from build123d import *

# Parameters (mm, degrees)
BOSS_EXTRUDE1_DEPTH        = 20
F_6_CLEARANCE_HOLE1_REACH  = 91.156
F_6_CLEARANCE_HOLE1_BORE_R = 1.89865
F_1_CLEARANCE_HOLE1_REACH  = 91.156
F_1_CLEARANCE_HOLE1_BORE_R = 1.0287
F_6_CLEARANCE_HOLE2_D      = 3.7973


with BuildPart() as part:
    # Sketch1 → Boss-Extrude1 (new body)
    with BuildSketch(Plane.XY):
        Polygon((30, 0), (0, 0), (0, 81.54), (30, 81.54), (30, 79.9525), (1.5875, 79.9525), (1.5875, 1.5875), (30, 1.5875), align=None)
    extrude(amount=BOSS_EXTRUDE1_DEPTH)

    # #6 Clearance Hole1 bore → #6 Clearance Hole1 (cut, up to next)
    with BuildSketch(Plane(origin=(0, 81.54, 0), x_dir=(1, 0, 0), z_dir=(0, 1, 0)), mode=Mode.PRIVATE) as f_6_clearance_hole1_sk1:
        with Locations((5, -10)):
            Circle(F_6_CLEARANCE_HOLE1_BORE_R)
    f_6_clearance_hole1_tool1 = extrude(f_6_clearance_hole1_sk1.sketch, amount=-F_6_CLEARANCE_HOLE1_REACH, mode=Mode.PRIVATE) & part.part
    # #6 Clearance Hole1 bore → #6 Clearance Hole1 (cut, up to next)
    with BuildSketch(Plane(origin=(0, 81.54, 0), x_dir=(1, 0, 0), z_dir=(0, 1, 0)), mode=Mode.PRIVATE) as f_6_clearance_hole1_sk2:
        with Locations((25, -10)):
            Circle(F_6_CLEARANCE_HOLE1_BORE_R)
    f_6_clearance_hole1_tool2 = extrude(f_6_clearance_hole1_sk2.sketch, amount=-F_6_CLEARANCE_HOLE1_REACH, mode=Mode.PRIVATE) & part.part
    add(f_6_clearance_hole1_tool1.solids().sort_by_distance((5, 81.54, 10))[0], mode=Mode.SUBTRACT)
    add(f_6_clearance_hole1_tool2.solids().sort_by_distance((25, 81.54, 10))[0], mode=Mode.SUBTRACT)

    # #1 Clearance Hole1 bore → #1 Clearance Hole1 (cut, up to next)
    with BuildSketch(Plane(origin=(0, 0, 0), x_dir=(-1, 0, 0), z_dir=(0, -1, 0)), mode=Mode.PRIVATE) as f_1_clearance_hole1_sk1:
        with Locations((-5.9, -10)):
            Circle(F_1_CLEARANCE_HOLE1_BORE_R)
    f_1_clearance_hole1_tool1 = extrude(f_1_clearance_hole1_sk1.sketch, amount=-F_1_CLEARANCE_HOLE1_REACH, mode=Mode.PRIVATE) & part.part
    # #1 Clearance Hole1 bore → #1 Clearance Hole1 (cut, up to next)
    with BuildSketch(Plane(origin=(0, 0, 0), x_dir=(-1, 0, 0), z_dir=(0, -1, 0)), mode=Mode.PRIVATE) as f_1_clearance_hole1_sk2:
        with Locations((-24.1, -10)):
            Circle(F_1_CLEARANCE_HOLE1_BORE_R)
    f_1_clearance_hole1_tool2 = extrude(f_1_clearance_hole1_sk2.sketch, amount=-F_1_CLEARANCE_HOLE1_REACH, mode=Mode.PRIVATE) & part.part
    add(f_1_clearance_hole1_tool1.solids().sort_by_distance((5.9, 0, 10))[0], mode=Mode.SUBTRACT)
    add(f_1_clearance_hole1_tool2.solids().sort_by_distance((24.1, 0, 10))[0], mode=Mode.SUBTRACT)

    # #6 Clearance Hole2 (through all)
    with Locations(Plane.ZY):
        with Locations((10, 28.08)):
            Hole(F_6_CLEARANCE_HOLE2_D / 2)


solid = part.part
Model file for the job. Use its own axes, mm. A direction names the side the tool comes from. Coordinates: 2 decimals unless noted, no trailing zeros. Order: outer loops, then holes, each group sorted by start corner. A loop starts at its lowest first (then second) coordinate and runs counter-clockwise, first axis right, second up. Notation, with made-up numbers: (1, 20.25) -> (59, 20.25) arc R13 ccw to (59, 34.25) -> close; hole circle Ø1 at (79.25, -23.5). An arc over 180 degrees is marked (long way). Return JSON: item names as keys, results as strings. Group by question number.
Item 1: Pull direction X, two halves, no side cores. Call faces 4 (the cylindrical face through (4.95, 0.78, 10.39)), 5 (the cylindrical face through (6.02, 80.76, 8.4)), 6 (the flat face through (1.588, 41, 10)), 7 (the flat face through (16, 79.952, 10)): pulls with the +X half, pulls with the -X half, needs draft (parallel to the pull), parting line crosses it, or undercut.
Item 2: Saw through at C-C on z = 10. Write the cut outline in (x, y), then the cut area to 3 significant figures.
Item 3: Saw through at D-D on x = 24.1. Write the cut outline in (y, z), then the cut area to 3 significant figures.
Item 4: Wall check: line 1 along X through (y, z) = (0.5, 10); line 2 along X through (y, z) = (80.7, 10); line 3 along Z through (x, y) = (5, 80.6). Give the ranges that are in metal, low to high. Write a range as [from, to].
Item 5: Tool access for faces 1 (the cylindrical face through (0.805, 26.226, 10.412)), 2 (the flat face through (16, 1.588, 10)), 3 (the cylindrical face through (26.8, 80.8, 9.4)): list every direction of +Z, -Z, +X, -X, +Y, -Y with a clear straight run to the whole face (end or side of a thin tool).
Item 6: Saw through at A-A on x = 14.5. Write the cut outline in (y, z), then the cut area to 3 significant figures.
Item 7: Saw through at B-B on z = 2. Write the cut outline in (x, y).
Item 8: Flat gauge pins, fed straight in: P1, Ø6, axis at y = 26, z = 6.5, coming from the +X side; P2, Ø2.5, axis at x = 5, z = 10, coming from the -Y side. Where does each tip first touch, or does it go through?
Values found:
{
 "1": {"face 4": "undercut", "face 5": "undercut", "face 6": "pulls with the +X half", "face 7": "needs draft"},
 "2": {"outline": "(0, 0) -> (4.87, 0) -> (4.87, 1.59) -> (1.59, 1.59) -> (1.59, 26.18) -> (0, 26.18) -> close; (0, 29.98) -> (1.59, 29.98) -> (1.59, 79.95) -> (3.1, 79.95) -> (3.1, 81.54) -> (0, 81.54) -> close; (6.9, 79.95) -> (23.1, 79.95) -> (23.1, 81.54) -> (6.9, 81.54) -> close; (6.93, 0) -> (23.07, 0) -> (23.07, 1.59) -> (6.93, 1.59) -> close; (25.13, 0) -> (30, 0) -> (30, 1.59) -> (25.13, 1.59) -> close; (26.9, 79.95) -> (30, 79.95) -> (30, 81.54) -> (26.9, 81.54) -> close", "area": "195 mm2"},
 "3": {"outline": "(0, 0) -> (1.59, 0) -> (1.59, 8.97) -> (0, 8.97) -> close; (0, 11.03) -> (1.59, 11.03) -> (1.59, 20) -> (0, 20) -> close; (79.95, 0) -> (81.54, 0) -> (81.54, 8.33) -> (79.95, 8.33) -> close; (79.95, 11.67) -> (81.54, 11.67) -> (81.54, 20) -> (79.95, 20) -> close", "area": "54.9 mm2"},
 "4": {"line 1": "x = [0, 4.87], [6.93, 23.07], [25.13, 30]", "line 2": "x = [0, 3.1], [6.9, 23.1], [26.9, 30]", "line 3": "z = [0, 8.1], [11.9, 20]"},
 "5": {"face 1": "+X, -X", "face 2": "+Z, -Z, +X", "face 3": "+Y"},
 "6": {"outline": "(0, 0) -> (1.59, 0) -> (1.59, 20) -> (0, 20) -> close; (79.95, 0) -> (81.54, 0) -> (81.54, 20) -> (79.95, 20) -> close", "area": "63.5 mm2"},
 "7": {"outline": "(0, 0) -> (30, 0) -> (30, 1.59) -> (1.59, 1.59) -> (1.59, 79.95) -> (30, 79.95) -> (30, 81.54) -> (0, 81.54) -> close"},
 "8": {"P1": "stops at x = 1.59", "P2": "stops at y = 0"}
}
